Here's how the part is built. I have some questions about the finished solid (model axes, mm). A direction names the side the tool comes from. Coordinates: 2 decimals unless noted, no trailing zeros. Order: outer loops, then holes, each group sorted by start corner. A loop starts at its lowest first (then second) coordinate and runs counter-clockwise, first axis right, second up. Notation, with made-up numbers: (27.5, 63.25) -> (68.5, 63.25) arc R29 ccw to (68.5, 98.25) -> close; hole circle Ø4 at (26, -4). An arc over 180 degrees is marked (long way). One line per item, written item: value. Start each with the question number.
```python
from build123d import *

# Parameters (mm, degrees)
F0_W     = 3
F0_H     = 3
F0_W_2   = 10
F1_DEPTH = 3
F2_W     = 10
F2_H     = 1.5
F3_DEPTH = 25


with BuildPart() as f1:
    # F0 (on Right) → F1 (new body)
    with BuildSketch(Plane.YZ):
        Polygon((-30, 11.18364), (-40, 11.18364), (-40, 5.22664), (-40, 2.22664), (-40, -0.77336), (-40, -3.77336), (-40, -6.77336), (-40, -9.77336), (-40, -11.18364), (-30, -11.18364), (-20, -11.18364), (-10, -11.18364), (0, -11.18364), (10, -11.18364), (20, -11.18364), (30, -11.18364), (40, -11.18364), (40, 11.18364), (30, 11.18364), (20, 11.18364), (10, 11.18364), (0, 11.18364), (-10, 11.18364), (-20, 11.18364), align=None)
        with Locations((-41.5, -8.27336)):
            Rectangle(F0_W, F0_H)
        with Locations((-41.5, 3.72664)):
            Rectangle(F0_W, F0_H)
        with Locations((-25, -12.68364)):
            Rectangle(F0_W_2, F0_H)
        with Locations((-25, 12.68364)):
            Rectangle(F0_W_2, F0_H)
        with Locations((-41.5, -2.27336)):
            Rectangle(F0_W, F0_H)
        with Locations((-5, -12.68364)):
            Rectangle(F0_W_2, F0_H)
        with Locations((-5, 12.68364)):
            Rectangle(F0_W_2, F0_H)
        with Locations((15, 12.68364)):
            Rectangle(F0_W_2, F0_H)
        with Locations((15, -12.68364)):
            Rectangle(F0_W_2, F0_H)
        with Locations((35, 12.68364)):
            Rectangle(F0_W_2, F0_H)
        with Locations((35, -12.68364)):
            Rectangle(F0_W_2, F0_H)
        with Locations((-25, -15.68364)):
            Rectangle(F0_W_2, F0_H)
        with Locations((-5, -15.68364)):
            Rectangle(F0_W_2, F0_H)
        with Locations((15, -15.68364)):
            Rectangle(F0_W_2, F0_H)
        with Locations((35, -15.68364)):
            Rectangle(F0_W_2, F0_H)
        with Locations((-35, -12.68364)):
            Rectangle(F0_W_2, F0_H)
        with Locations((-15, -12.68364)):
            Rectangle(F0_W_2, F0_H)
        with Locations((5, -12.68364)):
            Rectangle(F0_W_2, F0_H)
        with Locations((25, -12.68364)):
            Rectangle(F0_W_2, F0_H)
    extrude(amount=F1_DEPTH)

    # F2 (on face) → F3 (cut)
    with BuildSketch(Plane.YZ.offset(3)):
        with Locations((-25, -16.43364)):
            Rectangle(F2_W, F2_H)
        with Locations((-5, -16.43364)):
            Rectangle(F2_W, F2_H)
    extrude(amount=-F3_DEPTH, mode=Mode.SUBTRACT)


solid = f1.part
```
Q1. Imagine slicing it at A-A (y = -37). Write out the boundary of the cut face in (x, z), plus the area to 3 significant figures.
Q2. If we mould it in two halves opening along Y, with no side actions, what happens to faces 1 (the face through (1, -42, -3.773)), 2 (the face through (1, -30, 13)), 3 (the face through (1, 20, 13))? For each: +Y half, -Y half, draft (parallel to the pull), parting line (faces both ways), or undercut.
Q3. For P1, Ø1.5, axis at x = 2, z = 12, coming from the -Y side; P2, Ø0.9, axis at x = 1, y = -36.5, coming from the +Z side; P3, Ø1.5, axis at x = 2, y = -17.5, coming from the -Z side, each with a flat end and sliding along its axis, tell me the tip position at first contact or that it passes through.
Q4. I need wall thicknesses on line 1 (Z direction, x = 2.5, y = -23.5); line 2 (Y direction, x = 1.7, z = -11.5); line 3 (Z direction, x = 2.1, y = -38). Which ranges of each line are inside material? Lowest first, please.
Q5. For faces 4 (the face through (1, -10, -15)), 5 (the face through (1, -40, -12)), 6 (the face through (1, -42, 5.227)), 7 (the face through (1, -20, 13)), which set-ups out of +Z, -Z, +X, -X, +Y, -Y let a thin tool reach every point of the face, with its end or its side?
Q6. Imagine slicing it at B-B (z = 8.5). Write out the boundary of the cut face in (x, y).
Completed:
1. outline: (0, -14.18) -> (3, -14.18) -> (3, 11.18) -> (0, 11.18) -> close
1. area: 76.1 mm2
2. face 1: draft
2. face 2: -Y half
2. face 3: undercut
3. P1: stops at y = -30
3. P2: stops at z = 11.18
3. P3: stops at z = -14.18
4. line 1: z = -15.68 to 14.18
4. line 2: y = -40 to 40
4. line 3: z = -14.18 to 11.18
5. face 4: -Z, +X, -X
5. face 5: -Z, +X, -X, -Y
5. face 6: +Z, +X, -X, -Y
5. face 7: +Z, +X, -X
6. outline: (0, -40) -> (3, -40) -> (3, 40) -> (0, 40) -> close
